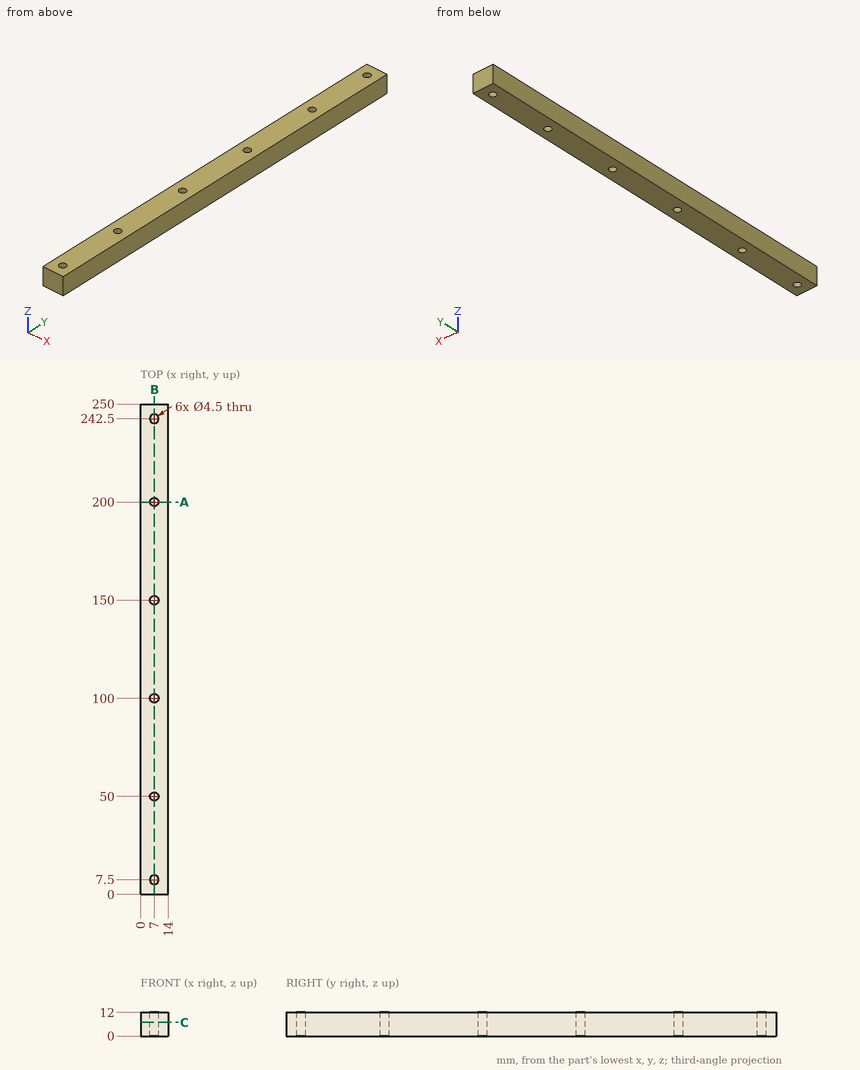
Verification items for this drawing (mm, ordinates from the low corner). Round coordinates to 2 decimals unless told otherwise and drop trailing zeros. Order: outer loops, then holes, each group sorted by start corner. A loop starts at its lowest first (then second) coordinate and runs counter-clockwise, first axis right, second up.
1) Depth check by flat-ended pin: pin 1 (3.5 mm diameter, centred on x = 7, y = 50, fed in from +Z). Enter the tip coordinate at first touch or a pass-through.
Geometry says:
pin 1: passes through
2) Cross-section at B-B, the plane x = 7. Record the cut outline in (y, z), plus the area to 3 significant figures.
Geometry says:
outline: (0, 0) - (5.25, 0) - (5.25, 12) - (0, 12) - close; (9.75, 0) - (47.75, 0) - (47.75, 12) - (9.75, 12) - close; (52.25, 0) - (97.75, 0) - (97.75, 12) - (52.25, 12) - close; (102.25, 0) - (147.75, 0) - (147.75, 12) - (102.25, 12) - close; (152.25, 0) - (197.75, 0) - (197.75, 12) - (152.25, 12) - close; (202.25, 0) - (240.25, 0) - (240.25, 12) - (202.25, 12) - close; (244.75, 0) - (250, 0) - (250, 12) - (244.75, 12) - close
area: 2,680 mm2
3) Cross-section at C-C, the plane z = 7. Record the cut outline in (x, y), plus the area to 3 significant figures.
Geometry says:
outline: (0, 0) - (14, 0) - (14, 250) - (0, 250) - close; hole circle Ø4.5 at (7, 7.5); hole circle Ø4.5 at (7, 50); hole circle Ø4.5 at (7, 100); hole circle Ø4.5 at (7, 150); hole circle Ø4.5 at (7, 200); hole circle Ø4.5 at (7, 242.5)
area: 3,400 mm2
4) Cross-section at A-A, the plane y = 200. Record the cut outline in (x, z), plus the area to 3 significant figures.
Geometry says:
outline: (0, 0) - (4.75, 0) - (4.75, 12) - (0, 12) - close; (9.25, 0) - (14, 0) - (14, 12) - (9.25, 12) - close
area: 114 mm2
